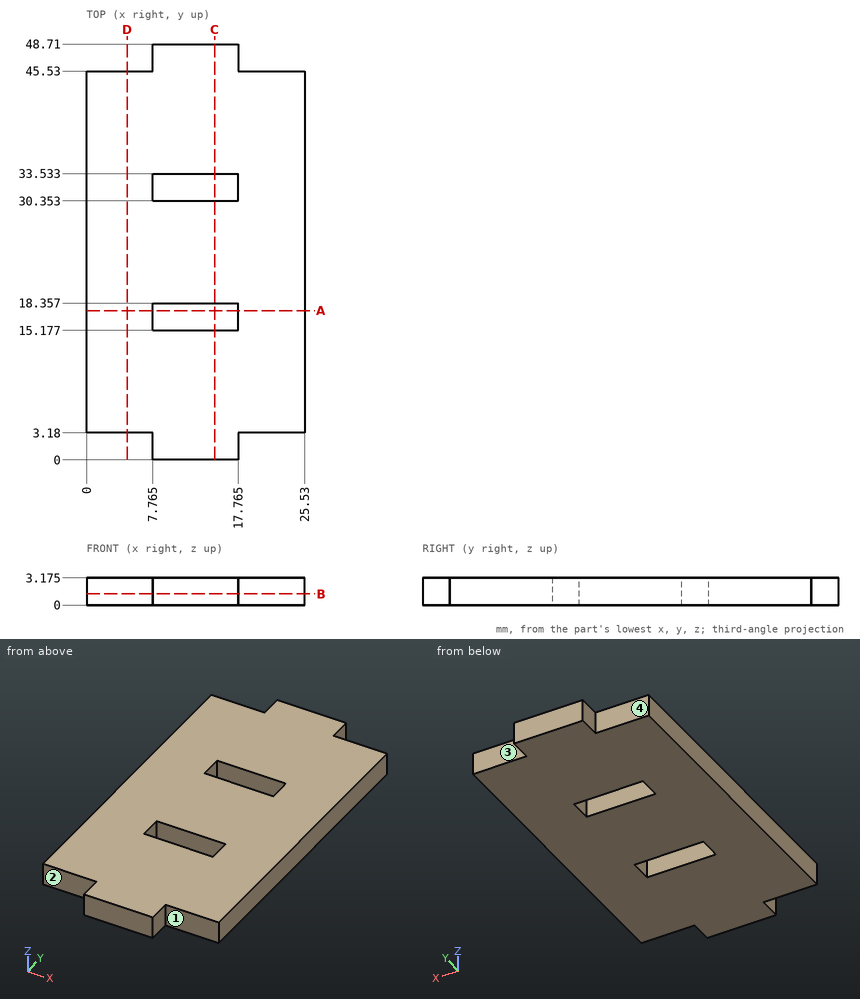
Geometry: see drawing. Coordinates: mm, zero at the bounding-box minimum. A direction names the side the tool comes from. Coordinates: 2 decimals unless noted, no trailing zeros. Order: outer loops, then holes, each group sorted by start corner. A loop starts at its lowest first (then second) coordinate and runs counter-clockwise, first axis right, second up. Notation, with made-up numbers: M 40,-37.75 L 77,-37.75 A29 cw 77,1.25 Z; hole C 87,0.25 d4. An arc over 180 degrees is marked long. Write item = value, one per line. Start each with the question number.
(1) Section B-B on z = 1.3. Output: boundary loops of the cut face in (x, y) (1 decimal), and give its area (3 significant figures).
(2) Section C-C on x = 15. Output: boundary loops of the cut face in (y, z) (1 decimal).
(3) Section D-D on x = 4.75. Output: boundary loops of the cut face in (y, z) (1 decimal).
(4) Line query: line 1 along Y through (x, z) = (15.25, 0.35); line 2 along X through (y, z) = (17, 1.1) (1 decimal); line 3 along Y through (x, z) = (5, 2.25). Output: solid intervals per line, ascending. Write a range as [from, to].
(5) Reachability of the marked faces 1, 2, 3 and 4 from +Z, -Z, +X, -X, +Y, -Y: full face, straight path, thin tool, end or side. Return the list, or none.
(6) Section A-A on y = 17.5. Output: boundary loops of the cut face in (x, z) (1 decimal), and give its area (3 significant figures).
(7) First-contact query: P1, Ø1, axis at y = 1, z = 1.5, coming from the -X side (3 decimals); P2, Ø1, axis at x = 21.5, z = 1.5, coming from the +Y side. Flat tips, straight axial feed; report the tip coordinate or a pass-through.
Result set:
q1.outline = M 0,3.2 L 7.8,3.2 L 7.8,0 L 17.8,0 L 17.8,3.2 L 25.5,3.2 L 25.5,45.5 L 17.8,45.5 L 17.8,48.7 L 7.8,48.7 L 7.8,45.5 L 0,45.5 Z; hole M 7.8,15.2 L 17.8,15.2 L 17.8,18.4 L 7.8,18.4 Z; hole M 7.8,30.4 L 17.8,30.4 L 17.8,33.5 L 7.8,33.5 Z
q1.area = 1,080 mm²
q2.outline = M 0,0 L 15.2,0 L 15.2,3.2 L 0,3.2 Z; M 18.4,0 L 30.4,0 L 30.4,3.2 L 18.4,3.2 Z; M 33.5,0 L 48.7,0 L 48.7,3.2 L 33.5,3.2 Z
q3.outline = M 3.2,0 L 45.5,0 L 45.5,3.2 L 3.2,3.2 Z
q4.line_1 = [0, 15.18], [18.36, 30.35], [33.53, 48.71]
q4.line_2 = [0, 7.8], [17.8, 25.5]
q4.line_3 = [3.18, 45.53]
q5.face_1 = +Z, -Z, +X, -Y
q5.face_2 = +Z, -Z, -X, -Y
q5.face_3 = +Z, -Z, +X, +Y
q5.face_4 = +Z, -Z, -X, +Y
q6.outline = M 0,0 L 7.8,0 L 7.8,3.2 L 0,3.2 Z; M 17.8,0 L 25.5,0 L 25.5,3.2 L 17.8,3.2 Z
q6.area = 49.3 mm²
q7.P1 = 7.765
q7.P2 = 45.53
